Geometry: final body of the model. Coordinates: model frame, mm. A direction names the side the tool comes from. Coordinates: 2 decimals unless noted, no trailing zeros. Loops run counter-clockwise (first coordinate to the right, second up) from the corner with the lowest first, then second, coordinate; pieces in that order, holes last. Notation, with made-up numbers: M 8.25,22.25 L 31.25,22.25 A24 ccw 31.25,44.25 Z; hole C -8.75,34 d9. An arc over 180 degrees is marked long. Write each question's results on one line, items separated by ' | '. Start each with the question number.
from build123d import *

# Parameters (mm, degrees)
F0_W     = 145
F0_H     = 165
F1_DEPTH = 4
F2_R     = 10
F4_DEPTH = 140
F5_R     = 5
F6_R     = 1
F7_R     = 1
F9_D     = 14
F11_D    = 11


with BuildPart() as f1:
    # F0 (on Top) → F1 (new body)
    with BuildSketch(Plane.XY):
        with Locations((-72.5, 41.823306)):
            Rectangle(F0_W, F0_H)
    extrude(amount=F1_DEPTH)

    # F2
    f2_edges = [f1.edges().sort_by_distance(p)[0] for p in [
        (0, -40.676694, 2),
        (0, 124.323306, 2),
        (-145, 124.323306, 2),
        (-145, -40.676694, 2),
    ]]
    fillet(f2_edges, radius=F2_R)

    # F3 (on face) → F4 (join)
    with BuildSketch(Plane.XY.offset(4)):
        Polygon((-19.5, 36.823306), (-19.5, 71.823306), (-125.5, 71.823306), (-125.5, 36.823306), (-123, 36.823306), (-123, 69.323306), (-22, 69.323306), (-22, 36.823306), align=None)
    extrude(amount=F4_DEPTH)

    # F5
    f5_edges = [f1.edges().sort_by_distance(p)[0] for p in [
        (-125.5, 71.823306, 74),
        (-19.5, 71.823306, 74),
    ]]
    fillet(f5_edges, radius=F5_R)

    # F6
    f6_edges = [f1.edges().sort_by_distance(p)[0] for p in [
        (-22, 69.323306, 74),
        (-123, 69.323306, 74),
    ]]
    fillet(f6_edges, radius=F6_R)

    # F7
    f7_edges = [f1.edges().sort_by_distance(p)[0] for p in [
        (-124.25, 36.823306, 144),
        (-20.75, 36.823306, 144),
    ]]
    fillet(f7_edges, radius=F7_R)

    # F9 (through all)
    with Locations(Plane.XY.offset(4)):
        with Locations((-22.5, 101.823306), (-72.5, 101.823306), (-122.5, 101.823306)):
            Hole(F9_D / 2)

    # F11 (through all)
    with Locations(Plane(origin=(0, 71.823306, 0), x_dir=(-1, 0, 0), z_dir=(0, 1, 0))):
        with Locations((102, 120), (43, 120), (43, 43.8), (102, 43.8)):
            Hole(F11_D / 2)


solid = f1.part
Item 1: Section A-A, the plane z = 43.8. Return loops of the section in (x, y), plus the area to 3 significant figures.
Item 2: Section C-C, the plane x = -43. Return loops of the section in (y, z), plus the area to 3 significant figures.
Item 3: Contact query for flat-ended pins moving along their axis: P1, Ø4, axis at x = -101.5, y = 83, coming from the +Z side; P2, Ø5, axis at x = -56.5, z = 62.5, coming from the +Y side; P3, Ø1.2, axis at x = -123.5, z = 84, coming from the -Y side. Output: stop coordinate, or through.
Item 4: Ray query, L1, parallel to Z at x = -102, y = 69.9; L2, parallel to X at y = 70, z = 43; L3, parallel to X at y = 53.5, z = 58. Return the intervals inside material, ascending. Write a range as [from, to].
Item 5: Set-up query: faces 5 (the flat face through (-74, 43, 4)), 6 (the cylindrical face through (-20.926, 70.32, 74.98)), 7 (the flat face through (-125.5, 52, 73)), 8 (the flat face through (-73, 69.323, 73)). Return all of +Z, -Z, +X, -X, +Y, -Y with unobstructed straight access to the full face (end or side cutting, diameter ignored); none if empty.
Item 6: Section D-D, the plane z = 13. Return loops of the section in (x, y), plus the area to 3 significant figures.
Item 7: Pull-direction query (X, two-part tool) for faces 1 (the flat face through (-73, -40.677, 2)), 2 (the cylindrical face through (-2.852, 121.316, 2.028)), 3 (the cylindrical face through (-123.996, 70.398, 74.98)), 4 (the cylindrical face through (-67.341, 106.554, 1.972)); classes: released by +X, released by -X, zero draft, split by the parting line, or undercut.
Item 8: Section B-B, the plane y = 53. Return loops of the section in (x, z), plus the area to 3 significant figures.
Solutions:
1) outline: M -125.5,36.82 L -123,36.82 L -123,68.32 A1 cw -122,69.32 L -107.5,69.32 L -107.5,71.82 L -120.5,71.82 A5 ccw -125.5,66.82 Z; M -96.5,69.32 L -48.5,69.32 L -48.5,71.82 L -96.5,71.82 Z; M -37.5,69.32 L -23,69.32 A1 cw -22,68.32 L -22,36.82 L -19.5,36.82 L -19.5,66.82 A5 ccw -24.5,71.82 L -37.5,71.82 Z | area: 362 mm²
2) outline: M -40.68,0 L 124.32,0 L 124.32,4 L 71.82,4 L 71.82,38.3 L 69.32,38.3 L 69.32,4 L -40.68,4 Z; M 69.32,49.3 L 71.82,49.3 L 71.82,114.5 L 69.32,114.5 Z; M 69.32,125.5 L 71.82,125.5 L 71.82,144 L 69.32,144 Z | area: 955 mm²
3) P1: stops at z = 4 | P2: stops at y = 71.82 | P3: stops at y = 36.82
4) L1: z = [0, 38.3], [49.3, 114.5], [125.5, 144] | L2: x = [-124.36, -107.44], [-96.56, -48.44], [-37.56, -20.64] | L3: x = [-125.5, -123], [-22, -19.5]
5) face 5: +Z | face 6: +Z, +X, +Y | face 7: +Z, -X, +Y, -Y | face 8: +Z, -Y
6) outline: M -125.5,36.82 L -123,36.82 L -123,68.32 A1 cw -122,69.32 L -23,69.32 A1 cw -22,68.32 L -22,36.82 L -19.5,36.82 L -19.5,66.82 A5 ccw -24.5,71.82 L -120.5,71.82 A5 ccw -125.5,66.82 Z | area: 417 mm²
7) face 1: zero draft | face 2: released by +X | face 3: released by -X | face 4: undercut
8) outline: M -145,0 L 0,0 L 0,4 L -19.5,4 L -19.5,144 L -22,144 L -22,4 L -123,4 L -123,144 L -125.5,144 L -125.5,4 L -145,4 Z | area: 1,280 mm²
